Answer from the drawing. Dimensions are ordinates in mm from the lowest x, y and z of the part. Coordinates: 2 decimals unless noted, no trailing zeros. Write each loop counter-clockwise with the first axis right and the second up, starting at its lowest first coordinate (ties: lowest second). Pieces come first, ordered by that corner, then holes.
1) The part is cut by section A-A (z = 7.5). Determine the outline of the cut face in (x, y).
2) The part is cut by section B-B (x = 120). Determine the outline of the cut face in (y, z) (3 decimals).
3) The part is cut by section C-C (y = 7). Determine the outline of the cut face in (x, z) (3 decimals).
4) Find the intervals of material crossed by line 1 (Y direction, x = 202.5, z = 4.25); line 2 (X direction, y = 10.5, z = 7.75); line 3 (Z direction, x = 218, y = 16) (3 decimals), in increasing order.
5) Determine the mould class of the marked faces 1, 2 and 3 for opening direction Y: +Y half, -Y half, draft (parallel to the pull), parting line (faces both ways), or undercut.
6) Each of these flat-tipped pins is pushed along its axis until it touches: pin 1 Ø3 at (x, y) = (154, 23) entering from -Z (3 decimals); pin 2 Ø10.5 at (y, z) = (42, 2.5) entering from -X; pin 3 Ø5 at (y, z) = (8, 5) entering from +X. Where does it stop, or does it pass through?
7) The part is cut by section D-D (y = 16.5). Determine the outline of the cut face in (x, z) (3 decimals), then the cut area to 3 significant figures.
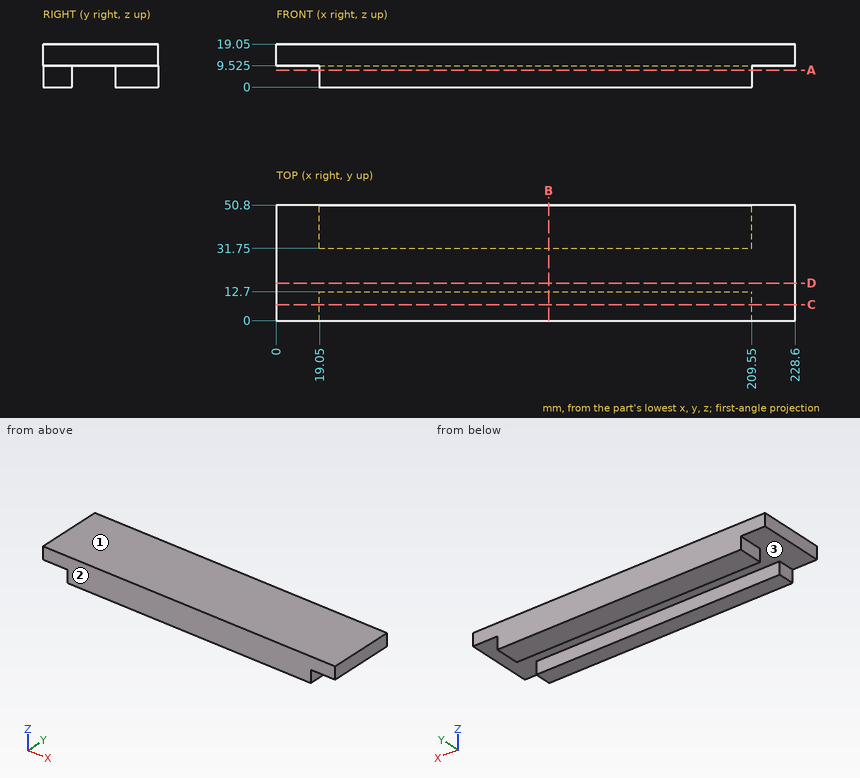
Reported:
1. outline: (19.05, 0) - (209.55, 0) - (209.55, 12.7) - (19.05, 12.7) - close; (19.05, 31.75) - (209.55, 31.75) - (209.55, 50.8) - (19.05, 50.8) - close
2. outline: (0, 0) - (12.7, 0) - (12.7, 9.525) - (31.75, 9.525) - (31.75, 0) - (50.8, 0) - (50.8, 19.05) - (0, 19.05) - close
3. outline: (0, 9.525) - (19.05, 9.525) - (19.05, 0) - (209.55, 0) - (209.55, 9.525) - (228.6, 9.525) - (228.6, 19.05) - (0, 19.05) - close
4. line 1: y = 0 to 12.7, 31.75 to 50.8
4. line 2: x = 19.05 to 209.55
4. line 3: z = 9.525 to 19.05
5. face 1: draft
5. face 2: -Y half
5. face 3: undercut
6. pin 1: stops at z = 9.525
6. pin 2: stops at x = 19.05
6. pin 3: stops at x = 209.55
7. outline: (0, 9.525) - (228.6, 9.525) - (228.6, 19.05) - (0, 19.05) - close
7. area: 2,180 mm2
